```python
from build123d import *

# Parameters (mm, degrees)
SKETCH1_W           = 14
SKETCH1_H           = 9
BOSS_EXTRUDE1_DEPTH = 2
SKETCH2_R           = 1.25
CUT_EXTRUDE1_DEPTH  = 2
SKETCH3_W           = 14
SKETCH3_H           = 2
BOSS_EXTRUDE2_DEPTH = 12
CUT_EXTRUDE2_DEPTH  = 12
SKETCH5_W           = 2
SKETCH5_H           = 5
BOSS_EXTRUDE3_DEPTH = 7
CUT_EXTRUDE3_DEPTH  = 14
SKETCH7_R           = 1.5
CUT_EXTRUDE4_DEPTH  = 2


with BuildPart() as part:
    # Sketch1 → Boss-Extrude1 (new body)
    with BuildSketch(Plane(origin=(0, 0, 0), x_dir=(1, 0, 0), z_dir=(0, 1, 0))):
        Rectangle(SKETCH1_W, SKETCH1_H)
    extrude(amount=BOSS_EXTRUDE1_DEPTH)

    # Sketch2 → Cut-Extrude1 (cut)
    with BuildSketch(Plane(origin=(0, 2, 0), x_dir=(1, 0, 0), z_dir=(0, 1, 0))):
        with Locations((-3, 1)):
            Circle(SKETCH2_R)
        with Locations((3, 1)):
            Circle(SKETCH2_R)
    extrude(amount=-CUT_EXTRUDE1_DEPTH, mode=Mode.SUBTRACT)

    # Sketch3 → Boss-Extrude2 (add)
    with BuildSketch(Plane(origin=(0, 2, 0), x_dir=(1, 0, 0), z_dir=(0, 1, 0))):
        with Locations((0, -3.5)):
            Rectangle(SKETCH3_W, SKETCH3_H)
    extrude(amount=BOSS_EXTRUDE2_DEPTH)

    # Sketch4 → Cut-Extrude2 (cut)
    with BuildSketch(Plane.XY.offset(4.5)):
        Polygon((-7, 7), (-4, 14), (-7, 14), align=None)
        Polygon((4, 14), (7, 7), (7, 14), align=None)
    extrude(amount=-CUT_EXTRUDE2_DEPTH, mode=Mode.SUBTRACT)

    # Sketch5 → Boss-Extrude3 (add)
    with BuildSketch(Plane(origin=(0, 0, 2.5), x_dir=(-1, 0, 0), z_dir=(0, 0, -1))):
        with Locations((-6, 4.5)):
            Rectangle(SKETCH5_W, SKETCH5_H)
        with Locations((6, 4.5)):
            Rectangle(SKETCH5_W, SKETCH5_H)
    extrude(amount=BOSS_EXTRUDE3_DEPTH)

    # Sketch6 → Cut-Extrude3 (cut)
    with BuildSketch(Plane(origin=(7, 0, 0), x_dir=(0, 0, -1), z_dir=(1, 0, 0))):
        Polygon((-2.5, 7), (4.5, 2), (4.5, 7), align=None)
    extrude(amount=-CUT_EXTRUDE3_DEPTH, mode=Mode.SUBTRACT)

    # Sketch7 → Cut-Extrude4 (cut)
    with BuildSketch(Plane.XY.offset(4.5)):
        with Locations((0, 8)):
            Circle(SKETCH7_R)
    extrude(amount=-CUT_EXTRUDE4_DEPTH, mode=Mode.SUBTRACT)


solid = part.part
```
Source: CAD feature listing. Evaluate the final solid. Frame: model axes, mm. A direction names the side the tool comes from. Round coordinates to 2 decimals unless told otherwise and drop trailing zeros. Loops run counter-clockwise (first coordinate to the right, second up) from the corner with the lowest first, then second, coordinate; pieces in that order, holes last.
1. Contact query for flat-ended pins moving along their axis: pin 1 (2 mm diameter, centred on x = 3, z = -1, fed in from +Y); pin 2 (3.5 mm diameter, centred on x = -1, y = 7.5, fed in from -Z). Output: stop coordinate, or through.
2. Section query C-C on y = 8. Output: boundary loops of the cut face in (x, z), and give its area (3 significant figures).
3. Section query A-A on z = -1. Output: boundary loops of the cut face in (x, y), and give its area (3 significant figures).
4. Access query for faces 4 (the flat face through (0, 14, 3)), 5 (the flat face through (5, 4, 0)). Directions: +Z, -Z, +X, -X, +Y, -Y. A direction counts if a zero-diameter tool reaches every point of the face in a straight line with its end or side. Return the directions, or none.
5. Mould query, pull axis Y, two halves, no side actions, for faces 1 (the flat face through (6, 4.5, -1)), 2 (the cylindrical face through (-0.325, 6.536, 3.514)), 3 (the flat face through (-2, 8, 2.5)). Classes: released by +Y, released by -Y, zero draft, split by the parting line, or undercut.
6. Ray query, L1, parallel to X at y = 0.5, z = -1; L2, parallel to Z at x = 3, y = 0.95; L3, parallel to Y at x = -4.25, z = 2. Return the intervals inside material, ascending.
7. Section query B-B on x = -3. Output: boundary loops of the cut face in (y, z), and give its area (3 significant figures).
8. Section query D-D on y = 6. Output: boundary loops of the cut face in (x, z).
Answers below:
1. pin 1: passes through
1. pin 2: stops at z = 2.5
2. outline: (-6.57, 2.5) - (-1.5, 2.5) - (-1.5, 4.5) - (-6.57, 4.5) - close; (1.5, 2.5) - (6.57, 2.5) - (6.57, 4.5) - (1.5, 4.5) - close
2. area: 20.3 mm2
3. outline: (-7, 0) - (-4.25, 0) - (-4.25, 2) - (-5, 2) - (-5, 4.5) - (-7, 4.5) - close; (-1.75, 0) - (1.75, 0) - (1.75, 2) - (-1.75, 2) - close; (4.25, 0) - (7, 0) - (7, 4.5) - (5, 4.5) - (5, 2) - (4.25, 2) - close
3. area: 28.0 mm2
4. face 4: +Z, -Z, +X, -X, +Y
4. face 5: -Z, +Y
5. face 1: released by +Y
5. face 2: undercut
5. face 3: zero draft
6. L1: x = -7 to -4.25, -1.75 to 1.75, 4.25 to 7
6. L2: z = -4.5 to -2.25, 0.25 to 4.5
6. L3: y = 0 to 2
7. outline: (0, -4.5) - (2, -4.5) - (2, -2.25) - (0, -2.25) - close; (0, 0.25) - (2, 0.25) - (2, 2.5) - (14, 2.5) - (14, 4.5) - (0, 4.5) - close
7. area: 37.0 mm2
8. outline: (-7, 1.1) - (-5, 1.1) - (-5, 2.5) - (5, 2.5) - (5, 1.1) - (7, 1.1) - (7, 4.5) - (-7, 4.5) - close
